from build123d import *

# Parameters (mm, degrees)
ESQUISSE1_W        = 140
ESQUISSE1_H        = 30
ESQUISSE1_R        = 1.6
BOSS_EXTRU_1_DEPTH = 3
ESQUISSE2_R        = 2.15
ESQUISSE2_R_2      = 1.6
BOSS_EXTRU_2_DEPTH = 2
CHANFREIN1_SIZE    = 0.2
CHANFREIN2_SIZE    = 1.5
CONG_1_R           = 1


with BuildPart() as part:
    # Esquisse1 → Boss.-Extru.1 (new body)
    with BuildSketch(Plane(origin=(0, 0, 0), x_dir=(1, 0, 0), z_dir=(0, 1, 0))):
        with Locations((70, 15)):
            Rectangle(ESQUISSE1_W, ESQUISSE1_H)
        with Locations(Location((4, 3.5, 0), (0, 0, 270))):
            Circle(ESQUISSE1_R, mode=Mode.SUBTRACT)
        with Locations(Location((26, 26.5, 0), (0, 0, 270))):
            Circle(ESQUISSE1_R, mode=Mode.SUBTRACT)
        with Locations(Location((114, 3.5, 0), (0, 0, 270))):
            Circle(ESQUISSE1_R, mode=Mode.SUBTRACT)
        with Locations(Location((136, 26.5, 0), (0, 0, 270))):
            Circle(ESQUISSE1_R, mode=Mode.SUBTRACT)
    extrude(amount=BOSS_EXTRU_1_DEPTH)

    # Esquisse2 → Boss.-Extru.2 (add)
    # profile 1 of 4: a face of its own
    with BuildSketch(Plane(origin=(0, 3, 0), x_dir=(1, 0, 0), z_dir=(0, 1, 0))):
        with Locations(Location((4, 3.5, 0), (0, 0, 270))):
            Circle(ESQUISSE2_R)
        with Locations(Location((4, 3.5, 0), (0, 0, 270))):
            Circle(ESQUISSE2_R_2, mode=Mode.SUBTRACT)
    # profile 2 of 4: a face of its own
    with BuildSketch(Plane(origin=(0, 3, 0), x_dir=(1, 0, 0), z_dir=(0, 1, 0))):
        with Locations(Location((26, 26.5, 0), (0, 0, 270))):
            Circle(ESQUISSE2_R)
        with Locations(Location((26, 26.5, 0), (0, 0, 270))):
            Circle(ESQUISSE2_R_2, mode=Mode.SUBTRACT)
    # profile 3 of 4: a face of its own
    with BuildSketch(Plane(origin=(0, 3, 0), x_dir=(1, 0, 0), z_dir=(0, 1, 0))):
        with Locations(Location((114, 3.5, 0), (0, 0, 270))):
            Circle(ESQUISSE2_R)
        with Locations(Location((114, 3.5, 0), (0, 0, 270))):
            Circle(ESQUISSE2_R_2, mode=Mode.SUBTRACT)
    # profile 4 of 4: a face of its own
    with BuildSketch(Plane(origin=(0, 3, 0), x_dir=(1, 0, 0), z_dir=(0, 1, 0))):
        with Locations(Location((136, 26.5, 0), (0, 0, 270))):
            Circle(ESQUISSE2_R)
        with Locations(Location((136, 26.5, 0), (0, 0, 270))):
            Circle(ESQUISSE2_R_2, mode=Mode.SUBTRACT)
    extrude(amount=BOSS_EXTRU_2_DEPTH)

    # Chanfrein1
    chanfrein1_edges = [part.edges().sort_by_distance(p)[0] for p in [
        (4, 5, -5.65),
        (4, 3, -5.65),
        (26, 5, -28.65),
        (26, 3, -28.65),
        (114, 5, -5.65),
        (114, 3, -5.65),
        (136, 5, -28.65),
        (136, 3, -28.65),
    ]]
    chamfer(chanfrein1_edges, length=CHANFREIN1_SIZE)

    # Chanfrein2
    chanfrein2_edges = [part.edges().sort_by_distance(p)[0] for p in [
        (4, 0, -5.1),
        (26, 0, -28.1),
        (114, 0, -5.1),
        (136, 0, -28.1),
    ]]
    chamfer(chanfrein2_edges, length=CHANFREIN2_SIZE)

    # Congé1
    cong_1_edges = [part.edges().sort_by_distance(p)[0] for p in [
        (0, 1.5, -30),
        (140, 1.5, -30),
        (140, 1.5, 0),
        (0, 1.5, 0),
    ]]
    fillet(cong_1_edges, radius=CONG_1_R)


solid = part.part
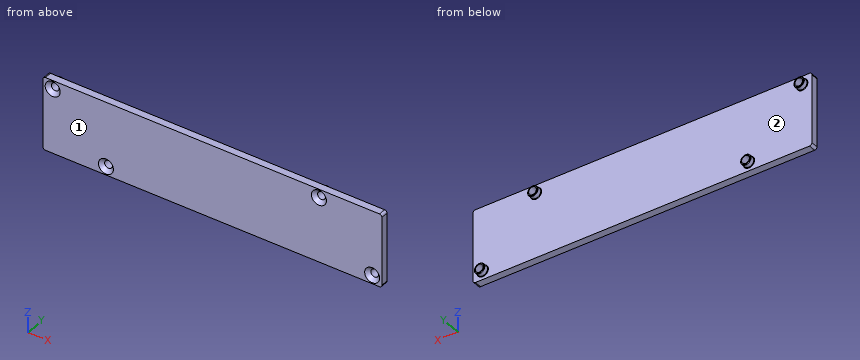
Model file for the job. Use its own axes, mm. Face numbers are marked on the shaded views. Give positions to 0.01 mm unless a question says otherwise; leave off trailing zeros. Loops run counter-clockwise (first coordinate to the right, second up) from the corner with the lowest first, then second, coordinate; pieces in that order, holes last. Notation, with made-up numbers: (50.5, 8.5) -> (100.5, 8.5) arc R14 cw to (100.5, 21.5) -> close; hole circle Ø3 at (-10, 10). An arc over 180 degrees is marked (long way). Use a Markdown table: item, result. Add a question column.
(1) Wall check: line 1 along X through (y, z) = (3.55, -26.5); line 2 along X through (y, z) = (3.75, -3.5); line 3 along X through (y, z) = (0.35, -27.75). Give the ranges that are in metal, low to high.
(2) Slice it at C-C on x = 69. List the corners of the cut face in (y, z).
(3) Mould opens along X. For the marked faces 1 and 2 say: +X half, -X half, draft (parallel to the pull), parting line (faces both ways), or undercut.
(4) Slice it at A-A on z = -3.5. Give the number of separate pieces and of enclosed holes in the cut face, and give its area (3 significant figures).
(5) Drop flat-ended pins along their axis: pin 1 Ø1.5 at (x, z) = (113.5, -16.5) entering from +Y; pin 2 Ø3.5 at (x, z) = (114, -3.5) entering from -Y. Give the stop position or say it passes through.
(6) Slice it at B-B on x = 114. List the corners of the cut face in (y, z).
Filled sheet:
| question | item | result |
|---|---|---|
| 1 | line 1 | 23.85 to 24.4, 27.6 to 28.15, 133.85 to 134.4, 137.6 to 138.15 |
| 1 | line 2 | 1.85 to 2.4, 5.6 to 6.15, 111.85 to 112.4, 115.6 to 116.15 |
| 1 | line 3 | 0 to 23.55, 28.45 to 133.55, 138.45 to 140 |
| 2 | outline | (0, -30) -> (3, -30) -> (3, 0) -> (0, 0) -> close |
| 3 | face 1 | draft |
| 3 | face 2 | undercut |
| 4 | separate pieces | 3 |
| 4 | enclosed holes | 0 |
| 4 | area | 401 mm2 |
| 5 | pin 1 | y = 3 |
| 5 | pin 2 | y = 1.35 |
| 6 | outline | (0, -30) -> (3, -30) -> (3, -5.85) -> (3.2, -5.65) -> (4.8, -5.65) -> (5, -5.45) -> (5, -5.1) -> (1.5, -5.1) -> (0, -6.6) -> close; (0, -0.4) -> (1.5, -1.9) -> (5, -1.9) -> (5, -1.55) -> (4.8, -1.35) -> (3.2, -1.35) -> (3, -1.15) -> (3, 0) -> (0, 0) -> close |
